Solid Edge part; units mm, degrees
sketch "Sketch1" plane through (0, 0, 0) normal (0, -1, 0) x (1, 0, 0)
  line L0 (-53.5, 0) -> (-53.5, 9)
  line L1 (-53.5, 9) -> (-52.5, 10)
  line L2 (-52.5, 10) -> (-3.5, 10)
  arc A0 (-1.5, 12) -> (-3.5, 10) centre (-3.5, 12) cw
  line L3 (-1.5, 12) -> (-1.5, 12.2)
  line L4 (-1, 12.7) -> (-1.5, 12.2)
  line L5 (-1, 12.7) -> (0, 12.7)
  line L6 (0, 12.7) -> (0, 0)
  line L7 (-53.5, 0) -> (0, 0)
  dimension "D1" = 53.5
  dimension "D2" = 3.5
revolve "RevolvedProtrusion1" add sketch "Sketch1" angle 360 about axis through (-60, 0, 0) along (1, 0, 0)
sketch "Sketch2" plane through (0, 0, 0) normal (0, 0, 1) x (1, 0, 0)
  line L0 (-53.5, 7) -> (-18.5, 7)
  arc A0 (-18.5, 7) -> (-5.2712, 12) centre (-18.5, 27) ccw
  line L1 (-5.2712, 12) -> (-53.5, 12)
  line L2 (-53.5, 12) -> (-53.5, 7)
extrude "Cutout1" cut sketch "Sketch2" along normal mid plane 5
hole "Thread_Hole" at (-53.5, 0, 0) direction (1, 0, 0) diameter 6.647 depth 30 tip angle 118 thread major 8 thread length 23
hole "Countersink_Hole" at (-53.5, 0, 0) direction (1, 0, 0) diameter 8.5 depth 5 countersink diameter 10 countersink angle 60
properties material "Steel"
The listing builds one solid part. Answer for the finished solid, in the listing's coordinates (mm). A direction names the side the tool comes from. Round coordinates to 2 decimals unless told otherwise and drop trailing zeros. Order: outer loops, then holes, each group sorted by start corner. A loop starts at its lowest first (then second) coordinate and runs counter-clockwise, first axis right, second up. Notation, with made-up numbers: (-40, 30) -> (14, 30) arc R16 ccw to (14, 53) -> close; hole circle Ø5 at (14.5, 62.5). An arc over 180 degrees is marked (long way). One line per item, written item: value.
Item 1: Find section A-A, the plane x = -43.5. Give the vertices of the cut face in (y, z), then the cut area to 3 significant figures.
Taken from the geometry:
outline: (7, -2.5) -> (7, 2.5) -> (9.68, 2.5) arc R10 ccw (long way) to (9.68, -2.5) -> close; hole circle Ø6.65 at (0, 0)
area: 265 mm2
Item 2: For a pull along Z with two mould halves and no side action, classify faces 4 (the flat face through (0, 0, 0)), 5 (the flat face through (-31, 8, -2.5)), 6 (the cylindrical face through (-27.66, -8.43, 5.38)) as released by +Z, released by -Z, zero draft, split by the parting line, or undercut.
Taken from the geometry:
face 4: zero draft
face 5: undercut
face 6: split by the parting line
Item 3: Straight lines are drawn through the part: L1, parallel to Y at x = -50.5, z = 0; L2, parallel to Y at x = -31.5, z = 0; L3, parallel to Z at x = -37.5, y = 0. For each, find the intervals that lie inside material, in ascending order.
Taken from the geometry:
L1: y = -10 to -4.25, 4.25 to 7
L2: y = -10 to -3.32, 3.32 to 7
L3: z = -10 to -3.32, 3.32 to 10
Item 4: Given P1, Ø1.5, axis at x = -18, z = -0.5, coming from the -Y side; P2, Ø0.8, axis at x = -33, y = 9, coming from the -Z side; P3, Ø6, axis at x = -22, z = -7.5, coming from the +Y side; P4, Ø8, axis at y = -1.5, z = 9, coming from the -X side, each flat-ended and moving along its own axis, determine where each tip first touches the part or whether it passes through.
Taken from the geometry:
P1: stops at y = -10
P2: stops at z = -5.1
P3: stops at y = 8.93
P4: stops at x = -53.5
Item 5: Find section C-C, the plane x = -17.5. Give the vertices of the cut face in (y, z), then the cut area to 3 significant figures.
Taken from the geometry:
outline: (7.03, -2.5) -> (7.03, 2.5) -> (9.68, 2.5) arc R10 ccw (long way) to (9.68, -2.5) -> close
area: 300 mm2
Item 6: For faces 1 (the cylindrical face through (-35.83, 1.27, 3.07)), 2 (the cylindrical face through (-0.49, 12.4, -2.75)), 3 (the cylindrical face through (-12.9, 7.8, 0)), determine the directions among +Z, -Z, +X, -X, +Y, -Y from which every point of the face is accessible in a straight line to the end or side of a thin tool.
Taken from the geometry:
face 1: -X
face 2: +X, -X
face 3: -X, +Y
Item 7: Find section B-B, the plane x = -5.5. Give the vertices of the cut face in (y, z), then the cut area to 3 significant figures.
Taken from the geometry:
outline: circle Ø20 at (0, 0)
area: 314 mm2
